```python
from build123d import *

# Parameters (mm, degrees)
BOSS_EXTRUDE1_DEPTH                               = 50.8
SKETCH3_R                                         = 3.2131
CUT_EXTRUDE1_DEPTH                                = 59.488981014
CSK_FOR_4_FLAT_HEAD_MACHINE_SCREW_100_D           = 3.2639
CSK_FOR_4_FLAT_HEAD_MACHINE_SCREW_100_CSINK_D     = 5.715
CSK_FOR_4_FLAT_HEAD_MACHINE_SCREW_100_CSINK_ANGLE = 100
Y_0_404_DIAMETER_HOLE1_D                          = 10.2616


with BuildPart() as part:
    # Sketch2 → Boss-Extrude1 (new body)
    with BuildSketch(Plane(origin=(0, 0, 0), x_dir=(0, 0, -1), z_dir=(1, 0, 0))):
        Polygon((0, 0), (0, 10.16), (13.97, 10.16), (13.97, 25.4), (25.4, 25.4), (25.4, 0), align=None)
    extrude(amount=BOSS_EXTRUDE1_DEPTH)

    # Sketch3 → Cut-Extrude1 (cut, through all)
    with BuildSketch(Plane.XY.offset(-13.97)):
        with Locations((12.7, 19.05)):
            Circle(SKETCH3_R)
    extrude(amount=-CUT_EXTRUDE1_DEPTH, mode=Mode.SUBTRACT)

    # CSK for #4 Flat Head Machine Screw (100)1 (through all)
    with Locations(Plane(origin=(0, 10.16, 0), x_dir=(1, 0, 0), z_dir=(0, 1, 0))):
        with Locations((6.35, 6.35), (28.575, 6.35)):
            CounterSinkHole(CSK_FOR_4_FLAT_HEAD_MACHINE_SCREW_100_D / 2, CSK_FOR_4_FLAT_HEAD_MACHINE_SCREW_100_CSINK_D / 2, counter_sink_angle=CSK_FOR_4_FLAT_HEAD_MACHINE_SCREW_100_CSINK_ANGLE)

    # Y (0.404) Diameter Hole1 (through all)
    with Locations(Plane(origin=(0, 0, -25.4), x_dir=(-1, 0, 0), z_dir=(0, 0, -1))):
        with Locations((-38.1, 19.05)):
            Hole(Y_0_404_DIAMETER_HOLE1_D / 2)


solid = part.part
```
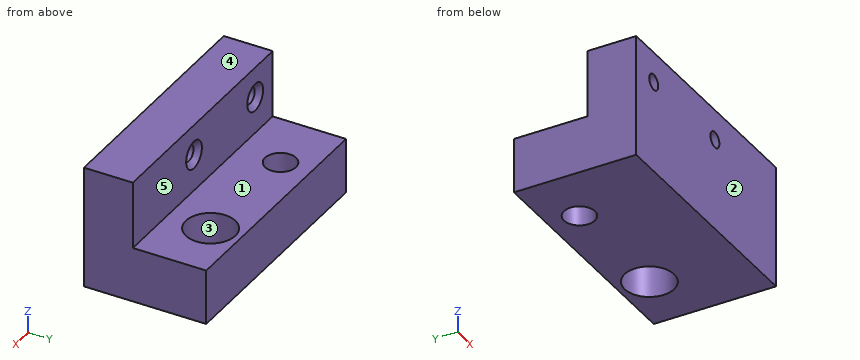
Input: part model. Units: mm. Frame: model coordinates. Face numbers are marked on the shaded views. A direction names the side the tool comes from. Coordinates: 2 decimals unless noted, no trailing zeros. Order: outer loops, then holes, each group sorted by start corner. A loop starts at its lowest first (then second) coordinate and runs counter-clockwise, first axis right, second up. Notation, with made-up numbers: (-37.75, 63) - (15.25, 63) arc R19 ccw to (15.25, 93) - close; hole circle Ø11 at (-28, 8.25). An arc over 180 degrees is marked (long way). Put each result on its own line as item: value.
1. Cut plane A-A on x = 38.1. Return the cut outline in (y, z).
Report:
outline: (0, -25.4) - (13.92, -25.4) - (13.92, -13.97) - (10.16, -13.97) - (10.16, 0) - (0, 0) - close; (24.18, -25.4) - (25.4, -25.4) - (25.4, -13.97) - (24.18, -13.97) - close
2. Cut plane C-C on z = -14.5. Return the cut outline in (x, y).
Report:
outline: (0, 0) - (50.8, 0) - (50.8, 25.4) - (0, 25.4) - close; hole circle Ø6.43 at (12.7, 19.05); hole circle Ø10.26 at (38.1, 19.05)
3. Cut plane D-D on x = 6.35. Return the cut outline in (y, z).
Report:
outline: (0, -25.4) - (25.4, -25.4) - (25.4, -13.97) - (10.16, -13.97) - (10.16, -9.21) - (9.13, -7.98) - (0, -7.98) - close; (0, -4.72) - (9.13, -4.72) - (10.16, -3.49) - (10.16, 0) - (0, 0) - close
4. Cut plane B-B on y = 19.05. Return the cut outline in (x, z).
Report:
outline: (0, -25.4) - (9.49, -25.4) - (9.49, -13.97) - (0, -13.97) - close; (15.91, -25.4) - (32.97, -25.4) - (32.97, -13.97) - (15.91, -13.97) - close; (43.23, -25.4) - (50.8, -25.4) - (50.8, -13.97) - (43.23, -13.97) - close
5. Draft query along Y for the marked faces 1, 2 and 3. Return one class per face: pulls with the +Y half, pulls with the -Y half, needs draft (parallel to the pull), parting line crosses it, or undercut.
Report:
face 1: needs draft
face 2: pulls with the -Y half
face 3: undercut
6. Line query: line 1 along X through (y, z) = (7, -6.35); line 2 along Y through (x, z) = (12.7, -17); line 3 along Z through (x, y) = (6.35, 6.5). Output: solid intervals per line, ascending.
Report:
line 1: x = 0 to 4.72, 7.98 to 26.94, 30.21 to 50.8
line 2: y = 0 to 15.84, 22.26 to 25.4
line 3: z = -25.4 to -7.98, -4.72 to 0
7. Reachability of the marked faces 4 and 5 from +Z, -Z, +X, -X, +Y, -Y: full face, straight path, thin tool, end or side. Return the list, or none.
Report:
face 4: +Z, +X, -X, +Y, -Y
face 5: +Z, +X, -X, +Y
8. Contact query for flat-ended pins moving along their axis: pin 1 Ø2 at (x, y) = (34.5, 5.5) entering from +Z; pin 2 Ø1.5 at (x, y) = (38, 21.5) entering from +Z; pin 3 Ø7 at (x, z) = (27, -4) entering from +Y; pin 4 Ø10.5 at (x, y) = (12.7, 19.05) entering from +Z. Output: stop coordinate, or through.
Report:
pin 1: stops at z = 0
pin 2: passes through
pin 3: stops at y = 10.16
pin 4: stops at z = -13.97
